For this review, take the finished solid that the model builds, in its own axes (mm). A direction names the side the tool comes from. Coordinates: 2 decimals unless noted, no trailing zeros. Loops run counter-clockwise (first coordinate to the right, second up) from the corner with the lowest first, then second, coordinate; pieces in that order, holes last. Notation, with made-up numbers: M 82,66 L 127,66 A23 cw 127,80 Z; hole C -0.75,51.5 d11. An arc over 180 degrees is marked long. Put each result on its own line as item: value.
```python
from build123d import *

# Parameters (mm, degrees)
IZIM1_W                 = 180
IZIM1_H                 = 176
TABAN_FLAN_1_DEPTH      = 4
RADYUS1_R               = 20
KES_EKSTR_ZYON1_DEPTH   = 10
IZIM7_W                 = 100
IZIM7_H                 = 116
KES_EKSTR_ZYON2_DEPTH   = 10
KENAR_FLAN_1_DEPTH      = 86.996406433
KENAR_FLAN_1_BEND_DEPTH = 87
IZIM14_R                = 4.25
KES_EKSTR_ZYON3_DEPTH   = 146
RADYUS2_R               = 10
IZIM15_W                = 125
IZIM15_H                = 33
SEKME1_DEPTH            = 4
RADYUS3_R               = 3
KES_EKSTR_ZYON4_DEPTH   = 1
KES_EKSTR_ZYON5_DEPTH   = 1
KES_EKSTR_ZYON6_DEPTH   = 10


# Sheet-metal steps are written as plain solids
with BuildPart() as part:
    # Çizim1 → Taban-Flanş1 (new body)
    with BuildSketch(Plane(origin=(0, 0, 0), x_dir=(1, 0, 0), z_dir=(0, 1, 0))):
        Rectangle(IZIM1_W, IZIM1_H)
    extrude(amount=-TABAN_FLAN_1_DEPTH)

    # Radyus1
    radyus1_edges = [part.edges().sort_by_distance(p)[0] for p in [
        (-90, -2, -88),
        (90, -2, -88),
        (90, -2, 88),
        (-90, -2, 88),
    ]]
    fillet(radyus1_edges, radius=RADYUS1_R)

    # Çizim6 → Kes-Ekstrüzyon1 (cut)
    with BuildSketch(Plane(origin=(0, 0, 0), x_dir=(1, 0, 0), z_dir=(0, 1, 0))):
        with BuildLine():
            Line((-71, -61.5), (-61, -61.5))
            ThreePointArc((-61, -61.5), (-53.5, -69), (-61, -76.5))
            Line((-61, -76.5), (-71, -76.5))
            ThreePointArc((-71, -76.5), (-78.5, -69), (-71, -61.5))
        make_face()
        with BuildLine():
            Line((-71, 76.5), (-61, 76.5))
            ThreePointArc((-61, 76.5), (-53.5, 69), (-61, 61.5))
            Line((-61, 61.5), (-71, 61.5))
            ThreePointArc((-71, 61.5), (-78.5, 69), (-71, 76.5))
        make_face()
        with BuildLine():
            Line((71, 61.5), (61, 61.5))
            ThreePointArc((61, 61.5), (53.5, 69), (61, 76.5))
            Line((61, 76.5), (71, 76.5))
            ThreePointArc((71, 76.5), (78.5, 69), (71, 61.5))
        make_face()
        with BuildLine():
            Line((71, -76.5), (61, -76.5))
            ThreePointArc((61, -76.5), (53.5, -69), (61, -61.5))
            Line((61, -61.5), (71, -61.5))
            ThreePointArc((71, -61.5), (78.5, -69), (71, -76.5))
        make_face()
    extrude(amount=-KES_EKSTR_ZYON1_DEPTH, mode=Mode.SUBTRACT)

    # Çizim7 → Kes-Ekstrüzyon2 (cut)
    with BuildSketch(Plane(origin=(0, 0, 0), x_dir=(1, 0, 0), z_dir=(0, 1, 0))):
        Rectangle(IZIM7_W, IZIM7_H)
    extrude(amount=-KES_EKSTR_ZYON2_DEPTH, mode=Mode.SUBTRACT)

    # Kenar-Flanş1 section (across the edge) → Kenar-Flanş1 (add)
    with BuildSketch(Plane(origin=(43.5, 0, 53), x_dir=(0, 0, 1), z_dir=(-1, 0, 0))):
        with BuildLine():
            Line((-4, 3.5), (-4, 25))
            Line((-4, 25), (0, 25))
            Line((0, 25), (0, 3.5))
            ThreePointArc((0, 3.5), (1.025126266, 1.025126266), (3.5, 0))
            Line((3.5, 0), (5, 0))
            Line((5, 0), (5, -4))
            Line((5, -4), (3.5, -4))
            ThreePointArc((3.5, -4), (-1.803300859, -1.803300859), (-4, 3.5))
        make_face()
    extrude(amount=KENAR_FLAN_1_DEPTH)

    # Kenar-Flanş1 section 2 (across the edge) → Kenar-Flanş1 bend (add)
    with BuildSketch(Plane(origin=(-43.5, 0, -53), x_dir=(0, 0, -1), z_dir=(1, 0, 0))):
        with BuildLine():
            Line((-4, 3.5), (-4, 25))
            Line((-4, 25), (0, 25))
            Line((0, 25), (0, 3.5))
            ThreePointArc((0, 3.5), (1.025126266, 1.025126266), (3.5, 0))
            Line((3.5, 0), (5, 0))
            Line((5, 0), (5, -4))
            Line((5, -4), (3.5, -4))
            ThreePointArc((3.5, -4), (-1.803300859, -1.803300859), (-4, 3.5))
        make_face()
    extrude(amount=KENAR_FLAN_1_BEND_DEPTH)

    # Çizim14 → Kes-Ekstrüzyon3 (cut)
    with BuildSketch(Plane(origin=(0, 0, -53), x_dir=(-1, 0, 0), z_dir=(0, 0, -1))):
        with Locations((-32.5, 16)):
            Circle(IZIM14_R)
        with Locations((32.5, 16)):
            Circle(IZIM14_R)
    extrude(amount=-KES_EKSTR_ZYON3_DEPTH, mode=Mode.SUBTRACT)

    # Radyus2
    radyus2_edges = [part.edges().sort_by_distance(p)[0] for p in [
        (43.5, 25, 51),
        (-43.496406433, 25, 51),
        (-43.5, 25, -51),
        (43.5, 25, -51),
    ]]
    fillet(radyus2_edges, radius=RADYUS2_R)

    # Çizim15 → Sekme1 (add)
    with BuildSketch(Plane(origin=(0, 0, 0), x_dir=(1, 0, 0), z_dir=(0, 1, 0))):
        Rectangle(IZIM15_W, IZIM15_H)
    extrude(amount=-SEKME1_DEPTH)

    # Radyus3
    radyus3_edges = [part.edges().sort_by_distance(p)[0] for p in [
        (-50, -2, 16.5),
        (-50, -2, -16.5),
        (50, -2, -16.5),
        (50, -2, 16.5),
    ]]
    fillet(radyus3_edges, radius=RADYUS3_R)

    # Çizim18 → Kes-Ekstrüzyon4 (cut)
    with BuildSketch(Plane(origin=(43.5, 0, 0), x_dir=(0, 0, -1), z_dir=(1, 0, 0))):
        with BuildLine():
            Line((53, 3.5), (49, 3.5))
            ThreePointArc((49, 3.5), (51.196699141, -1.803300859), (56.5, -4))
            Line((56.5, -4), (56.5, 0))
            ThreePointArc((56.5, 0), (54.025126266, 1.025126266), (53, 3.5))
        make_face()
        with BuildLine():
            Line((-49, 3.5), (-53, 3.5))
            ThreePointArc((-53, 3.5), (-54.025126266, 1.025126266), (-56.5, 0))
            Line((-56.5, 0), (-56.5, -4))
            ThreePointArc((-56.5, -4), (-51.196699141, -1.803300859), (-49, 3.5))
        make_face()
    extrude(amount=-KES_EKSTR_ZYON4_DEPTH, mode=Mode.SUBTRACT)

    # Çizim19 → Kes-Ekstrüzyon5 (cut)
    with BuildSketch(Plane.ZY.offset(43.5)):
        with BuildLine():
            Line((-49, 3.5), (-53, 3.5))
            ThreePointArc((-53, 3.5), (-54.025126266, 1.025126266), (-56.5, 0))
            Line((-56.5, 0), (-56.5, -4))
            ThreePointArc((-56.5, -4), (-51.196699141, -1.803300859), (-49, 3.5))
        make_face()
        with BuildLine():
            Line((53, 3.5), (49, 3.5))
            ThreePointArc((49, 3.5), (51.196699141, -1.803300859), (56.5, -4))
            Line((56.5, -4), (56.5, 0))
            ThreePointArc((56.5, 0), (54.025126266, 1.025126266), (53, 3.5))
        make_face()
    extrude(amount=-KES_EKSTR_ZYON5_DEPTH, mode=Mode.SUBTRACT)

    # Çizim20 → Kes-Ekstrüzyon6 (cut)
    with BuildSketch(Plane(origin=(0, 0, 0), x_dir=(1, 0, 0), z_dir=(0, 1, 0))):
        with BuildLine():
            Line((102, -7.5), (78, -7.5))
            ThreePointArc((78, -7.5), (70.5, 0), (78, 7.5))
            Line((78, 7.5), (102, 7.5))
            ThreePointArc((102, 7.5), (109.5, 0), (102, -7.5))
        make_face()
        with BuildLine():
            Line((-102, 7.5), (-78, 7.5))
            ThreePointArc((-78, 7.5), (-70.5, 0), (-78, -7.5))
            Line((-78, -7.5), (-102, -7.5))
            ThreePointArc((-102, -7.5), (-109.5, 0), (-102, 7.5))
        make_face()
    extrude(amount=-KES_EKSTR_ZYON6_DEPTH, mode=Mode.SUBTRACT)


solid = part.part
```
(1) Add section A-A (y = 9.5). Write out the cut boundary in (x, z).
Determined:
outline: M -43.5,-53 L 43.5,-53 L 43.5,-49 L -43.5,-49 Z; M -43.5,49 L 43.5,49 L 43.5,53 L -43.5,53 Z
(2) Add section B-B (x = 31). Write out the cut boundary in (y, z), plus the area to 3 significant figures.
Determined:
outline: M -4,-88 L 0,-88 L 0,-56.5 A3.5 cw 3.5,-53 L 12.02,-53 L 12.02,-49 L 3.5,-49 A7.5 ccw -4,-56.5 Z; M -4,-16.5 L 0,-16.5 L 0,16.5 L -4,16.5 Z; M -4,56.5 A7.5 ccw 3.5,49 L 12.02,49 L 12.02,53 L 3.5,53 A3.5 cw 0,56.5 L 0,88 L -4,88 Z; M 19.98,-53 L 25,-53 L 25,-49 L 19.98,-49 Z; M 19.98,49 L 25,49 L 25,53 L 19.98,53 Z
area: 561 mm^2
(3) Tool access review of faces 5 (the flat face through (-47, -2, 58)), 6 (the flat face through (43.5, 9, -51)), 7 (the flat face through (-42.5, 0, 53)), 8 (the cylindrical face through (36.746, 16.187, -51.028)), 9 (the flat face through (-84, -2, 7.5)): name each direction out of +Z, -Z, +X, -X, +Y, -Y from which nothing blocks a thin tool from reaching the whole face with its end or side.
Determined:
face 5: +Y, -Y
face 6: +Z, -Z, +X, +Y, -Y
face 7: -Y
face 8: +Z, -Z
face 9: -X, +Y, -Y
(4) For pin 1 (1.2 mm diameter, centred on x = -85.5, y = -3, fed in from -Z); pin 2 (12 mm diameter, centred on x = -38.5, z = -59.5, fed in from +Y); pin 3 (4.5 mm diameter, centred on y = 9.5, z = -50.5, fed in from +X), all flat-tipped, find the tip position at first contact; note any pin that passes through.
Determined:
pin 1: stops at z = -81.34
pin 2: stops at y = 1.7
pin 3: stops at x = 43.5
(5) Add section C-C (z = 0). Write out the cut boundary in (x, y), plus the area to 3 significant figures.
Determined:
outline: M -70.5,-4 L 70.5,-4 L 70.5,0 L -70.5,0 Z
area: 564 mm^2
(6) Draft analysis for pull direction X (two halves, no side actions). For faces 1 (the cylindrical face through (-70.5, -1.97, -0.16)), 2 (the cylindrical face through (-78.5, -1.97, -68.84)), 3 (the cylindrical face through (83.986, -2.028, 82.297)), 4 (the flat face through (84, -2, 7.5)), state which applies: +X half, -X half, draft (parallel to the pull), parting line (faces both ways), or undercut.
Determined:
face 1: -X half
face 2: undercut
face 3: +X half
face 4: draft
(7) Wall thickness on line 1 along Z through (x, y) = (46.5, -1.5); line 2 along Z through (x, y) = (2, 10.25); line 3 along Z through (x, y) = (-21.5, -2): over which ranges is each line inside the solid? List them lowest first. Write a range as [from, to].
Determined:
line 1: z = [-88, -58], [-16.5, 16.5], [58, 88]
line 2: z = [-53, -49], [49, 53]
line 3: z = [-88, -51.4], [-16.5, 16.5], [51.4, 88]
